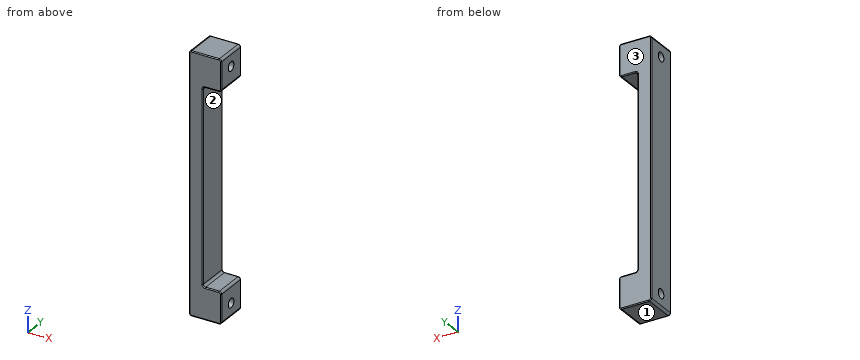
```python
from build123d import *

# Parameters (mm, degrees)
F0_R     = 1
F1_DEPTH = 7
F0_W     = 7
F0_H     = 42.2
F2_DEPTH = 3
F3_R     = 0.5
F4_R     = 0.2


with BuildPart() as f1:
    # F0 (on Right) → F1 (new body)
    with BuildSketch(Plane.YZ):
        Polygon((3.5, -22.5), (3.5, -21.1), (-3.5, -21.1), (-3.5, -22.5), (-3.5, -28), (3.5, -28), align=None)
        with Locations((0, -25)):
            Circle(F0_R, mode=Mode.SUBTRACT)
    extrude(amount=F1_DEPTH)



with BuildPart() as f1b:
    # F0 (on Right) → F1, piece 2 (new body)
    with BuildSketch(Plane.YZ):
        Polygon((3.5, 22.5), (3.5, 28), (-3.5, 28), (-3.5, 22.5), (-3.5, 21.1), (3.5, 21.1), align=None)
        with Locations((0, 25)):
            Circle(F0_R, mode=Mode.SUBTRACT)
    extrude(amount=F1_DEPTH)


with BuildPart() as f1_1:
    add(f1.part)

    add(f1b.part)  # F2 merges F1b
    # F0 (on Right) → F2 (join)
    with BuildSketch(Plane.YZ):
        Rectangle(F0_W, F0_H)
    extrude(amount=F2_DEPTH)

    # F3
    f3_edges = [f1_1.edges().sort_by_distance(p)[0] for p in [
        (7, 0, -21.1),
        (7, 0, -28),
        (7, 0, 21.1),
        (7, 0, 28),
        (0, 0, 28),
        (0, 0, -28),
        (3, 0, 21.1),
        (3, 0, -21.1),
    ]]
    fillet(f3_edges, radius=F3_R)

    # F4
    f4_edges = [f1_1.edges().sort_by_distance(p)[0] for p in [
        (3, 3.5, 0),
        (3, -3.5, 0),
        (3.5, 3.5, 28),
        (0.146447, 3.5, 27.853553),
        (6.853553, 3.5, 27.853553),
        (0, 3.5, 0),
        (7, 3.5, 24.55),
        (0.146447, 3.5, -27.853553),
        (6.853553, 3.5, 21.246447),
        (3.5, 3.5, -28),
        (5, 3.5, 21.1),
        (6.853553, 3.5, -27.853553),
        (3.146447, 3.5, 20.953553),
        (7, 3.5, -24.55),
        (6.853553, 3.5, -21.246447),
        (3.146447, 3.5, -20.953553),
        (5, 3.5, -21.1),
        (3.5, -3.5, 28),
        (0.146447, -3.5, 27.853553),
        (6.853553, -3.5, 27.853553),
        (0, -3.5, 0),
        (7, -3.5, 24.55),
        (0.146447, -3.5, -27.853553),
        (6.853553, -3.5, 21.246447),
        (3.5, -3.5, -28),
        (5, -3.5, 21.1),
        (6.853553, -3.5, -27.853553),
        (3.146447, -3.5, 20.953553),
        (7, -3.5, -24.55),
        (6.853553, -3.5, -21.246447),
        (3.146447, -3.5, -20.953553),
        (5, -3.5, -21.1),
    ]]
    fillet(f4_edges, radius=F4_R)


solid = f1_1.part
```
The model under review builds one solid part; all positions refer to its coordinate system, in mm. Face numbers are marked on the shaded views. Give positions to 0.01 mm unless a question says otherwise; leave off trailing zeros. Write each loop counter-clockwise with the first axis right and the second up, starting at its lowest first coordinate (ties: lowest second). Pieces come first, ordered by that corner, then holes. Notation, with made-up numbers: M 1.5,-1 L 13.5,-1 A21 ccw 13.5,35 Z; hole C -13,78 d9. An arc over 180 degrees is marked long. Answer in a Markdown table with one row per item.
Item 1: Add section C-C on y = 0.25. Give the boundary of the cut face in (x, z).
Check sheet entries:
| item | result |
|---|---|
| outline | M 0,-27.5 A0.5 ccw 0.5,-28 L 6.5,-28 A0.5 ccw 7,-27.5 L 7,-25.97 L 0,-25.97 Z; M 0,-24.03 L 7,-24.03 L 7,-21.6 A0.5 ccw 6.5,-21.1 L 3.5,-21.1 A0.5 cw 3,-20.6 L 3,20.6 A0.5 cw 3.5,21.1 L 6.5,21.1 A0.5 ccw 7,21.6 L 7,24.03 L 0,24.03 Z; M 0,25.97 L 7,25.97 L 7,27.5 A0.5 ccw 6.5,28 L 0.5,28 A0.5 ccw 0,27.5 Z |
Item 2: For P1, Ø3.5, axis at y = 1.5, z = -2.5, coming from the +X side, flat-tipped, find the tip position at first contact; note if it passes through.
Check sheet entries:
| item | result |
|---|---|
| P1 | x = 3 |
Item 3: Add section B-B on x = 2.25. Give the boundary of the cut face in (y, z), plus the area to 3 significant figures.
Check sheet entries:
| item | result |
|---|---|
| outline | M -3.5,-27.8 A0.2 ccw -3.3,-28 L 3.3,-28 A0.2 ccw 3.5,-27.8 L 3.5,27.8 A0.2 ccw 3.3,28 L -3.3,28 A0.2 ccw -3.5,27.8 Z; hole C 0,-25 d2; hole C 0,25 d2 |
| area | 386 mm2 |
Item 4: Add section A-A on z = -25. Give the boundary of the cut face in (x, y), plus the area to 3 significant figures.
Check sheet entries:
| item | result |
|---|---|
| outline | M 0,-3.3 A0.2 ccw 0.2,-3.5 L 6.8,-3.5 A0.2 ccw 7,-3.3 L 7,-1 L 0,-1 Z; M 0,1 L 7,1 L 7,3.3 A0.2 ccw 6.8,3.5 L 0.2,3.5 A0.2 ccw 0,3.3 Z |
| area | 35.0 mm2 |
Item 5: Add section D-D on y = 2.25. Give the boundary of the cut face in (x, z), plus the area to 3 significant figures.
Check sheet entries:
| item | result |
|---|---|
| outline | M 0,-27.5 A0.5 ccw 0.5,-28 L 6.5,-28 A0.5 ccw 7,-27.5 L 7,-21.6 A0.5 ccw 6.5,-21.1 L 3.5,-21.1 A0.5 cw 3,-20.6 L 3,20.6 A0.5 cw 3.5,21.1 L 6.5,21.1 A0.5 ccw 7,21.6 L 7,27.5 A0.5 ccw 6.5,28 L 0.5,28 A0.5 ccw 0,27.5 Z |
| area | 223 mm2 |
Item 6: For line 1 along Z through (x, y) = (2.25, 0); line 2 along Z through (x, y) = (4, 0); line 3 along Z through (x, y) = (5.5, -0.75), list the stretches that pass through material, from the lowest coordinate up.
Check sheet entries:
| item | result |
|---|---|
| line 1 | -28 to -26, -24 to 24, 26 to 28 |
| line 2 | -28 to -26, -24 to -21.1, 21.1 to 24, 26 to 28 |
| line 3 | -28 to -25.66, -24.34 to -21.1, 21.1 to 24.34, 25.66 to 28 |
Item 7: Draft analysis for pull direction Z (two halves, no side actions). For the marked faces 1, 2 and 3, state which applies: +Z half, -Z half, draft (parallel to the pull), parting line (faces both ways), or undercut.
Check sheet entries:
| item | result |
|---|---|
| face 1 | -Z half |
| face 2 | undercut |
| face 3 | draft |
